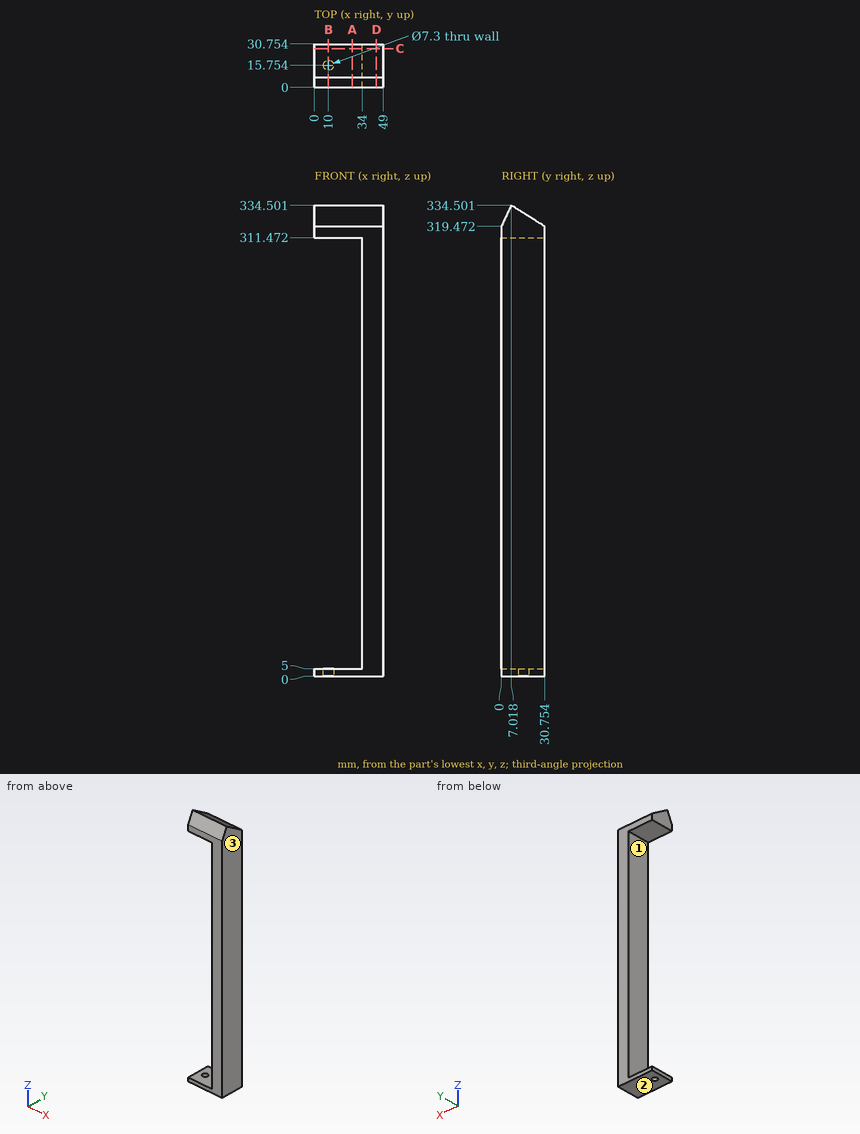
Can you work these out from the drawing? Everything is in mm from the part's minimum corner. Round coordinates to 2 decimals unless told otherwise and drop trailing zeros. Write each loop counter-clockwise with the first axis right and the second up, starting at its lowest first coordinate (ties: lowest second). Pieces come first, ordered by that corner, then holes.
1. I need wall thicknesses on L1, parallel to Y at x = 10, z = 3.5; L2, parallel to Z at x = 31.5, y = 17; L3, parallel to X at y = 25, z = 143. Which ranges of each line are inside material? Lowest first, please.
2. Suppose I cut it at B-B (x = 10). List the corners of the cut face in (y, z) for me, and give its area (3 significant figures).
3. Suppose I cut it at D-D (x = 44). List the corners of the cut face in (y, z) for me, and give its area (3 significant figures).
4. Suppose I cut it at A-A (x = 27). List the corners of the cut face in (y, z) for me, and give its area (3 significant figures).
5. If we mould it in two halves opening along Z, with no side actions, what happens to the marked faces 1, 2 and 3? For each: released by +Z, released by -Z, zero draft, split by the parting line, or undercut.
6. Suppose I cut it at C-C (y = 27.5). List the corners of the cut face in (x, z) for me.
7. Will these pins go through, and if not, where does the flat tip stop? pin 1 Ø1.5 at (y, z) = (25, 34) entering from -X; pin 2 Ø2 at (x, y) = (41, 17.5) entering from -Z; pin 3 Ø9.5 at (x, y) = (10, 15.75) entering from +Z.
Answer sheet:
1. L1: y = 0 to 12.1, 19.4 to 30.75
1. L2: z = 0 to 5, 311.47 to 328.18
1. L3: x = 34 to 49
2. outline: (0, 0) - (12.1, 0) - (12.1, 5) - (0, 5) - close; (0, 311.47) - (30.75, 311.47) - (30.75, 319.47) - (7.02, 334.5) - (0, 319.47) - close; (19.4, 0) - (30.75, 0) - (30.75, 5) - (19.4, 5) - close
2. area: 594 mm2
3. outline: (0, 0) - (30.75, 0) - (30.75, 319.47) - (7.02, 334.5) - (0, 319.47) - close
3. area: 10,100 mm2
4. outline: (0, 0) - (30.75, 0) - (30.75, 5) - (0, 5) - close; (0, 311.47) - (30.75, 311.47) - (30.75, 319.47) - (7.02, 334.5) - (0, 319.47) - close
4. area: 631 mm2
5. face 1: undercut
5. face 2: released by -Z
5. face 3: zero draft
6. outline: (0, 0) - (49, 0) - (49, 321.53) - (0, 321.53) - (0, 311.47) - (34, 311.47) - (34, 5) - (0, 5) - close
7. pin 1: stops at x = 34
7. pin 2: stops at z = 0
7. pin 3: stops at z = 331.98
